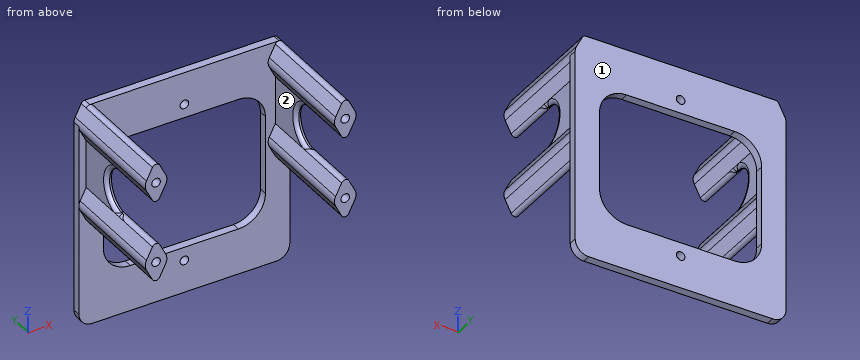
```python
from build123d import *

# Parameters (mm, degrees)
SKETCH1_R             = 1.6
BOSS_EXTRUDE1_DEPTH   = 40
BOSS_EXTRUDE1_2_DEPTH = 40
BOSS_EXTRUDE1_3_DEPTH = 40
BOSS_EXTRUDE1_4_DEPTH = 40
SKETCH2_R             = 1.6
BOSS_EXTRUDE2_DEPTH   = 3
SKETCH4_W             = 2.672170628
SKETCH4_H             = 17.636363636
BOSS_EXTRUDE3_DEPTH   = 20
SKETCH6_R             = 8
CUT_EXTRUDE2_DEPTH    = 99.18617902
FILLET1_R             = 1.5
BOSS_EXTRUDE4_START   = 20
SKETCH7_R             = 1.6
BOSS_EXTRUDE4_DEPTH   = 20


# Read off the part's stored shape, not the designer's step: Mirror2
with BuildPart() as part:
    # Sketch1 → Boss-Extrude1 (new body)
    with BuildSketch(Plane(origin=(0, 0, 0), x_dir=(1, 0, 0), z_dir=(0, 1, 0))):
        with BuildLine():
            Line((-1.336085314, 6.181818182), (-3.562894171, 1.818181818))
            ThreePointArc((-3.562894171, 1.818181818), (-4, 0), (-3.562894171, -1.818181818))
            Line((-3.562894171, -1.818181818), (-1.336085314, -6.181818182))
            ThreePointArc((-1.336085314, -6.181818182), (0, -7), (1.336085314, -6.181818182))
            Line((1.336085314, -6.181818182), (3.562894171, -1.818181818))
            ThreePointArc((3.562894171, -1.818181818), (4, 0), (3.562894171, 1.818181818))
            Line((3.562894171, 1.818181818), (1.336085314, 6.181818182))
            ThreePointArc((1.336085314, 6.181818182), (0, 7), (-1.336085314, 6.181818182))
        make_face()
        with Locations(Location((0, 0, 0), (0, 0, 270))):
            Circle(SKETCH1_R, mode=Mode.SUBTRACT)
    extrude(amount=BOSS_EXTRUDE1_DEPTH)



with BuildPart() as body_2:
    # Sketch1 → Boss-Extrude1 2 (new body)
    with BuildSketch(Plane(origin=(0, 0, 0), x_dir=(1, 0, 0), z_dir=(0, 1, 0))):
        with BuildLine():
            Line((68.663914686, 6.181818182), (66.437105829, 1.818181818))
            ThreePointArc((66.437105829, 1.818181818), (66, 0), (66.437105829, -1.818181818))
            Line((66.437105829, -1.818181818), (68.663914686, -6.181818182))
            ThreePointArc((68.663914686, -6.181818182), (70, -7), (71.336085314, -6.181818182))
            Line((71.336085314, -6.181818182), (73.562894171, -1.818181818))
            ThreePointArc((73.562894171, -1.818181818), (74, 0), (73.562894171, 1.818181818))
            Line((73.562894171, 1.818181818), (71.336085314, 6.181818182))
            ThreePointArc((71.336085314, 6.181818182), (70, 7), (68.663914686, 6.181818182))
        make_face()
        with Locations(Location((70, 0, 0), (0, 0, 270))):
            Circle(SKETCH1_R, mode=Mode.SUBTRACT)
    extrude(amount=BOSS_EXTRUDE1_2_DEPTH)


with BuildPart() as body_3:
    # Sketch1 → Boss-Extrude1 3 (new body)
    with BuildSketch(Plane(origin=(0, 0, 0), x_dir=(1, 0, 0), z_dir=(0, 1, 0))):
        with BuildLine():
            Line((68.663914686, -23.818181818), (66.437105829, -28.181818182))
            ThreePointArc((66.437105829, -28.181818182), (66, -30), (66.437105829, -31.818181818))
            Line((66.437105829, -31.818181818), (68.663914686, -36.181818182))
            ThreePointArc((68.663914686, -36.181818182), (70, -37), (71.336085314, -36.181818182))
            Line((71.336085314, -36.181818182), (73.562894171, -31.818181818))
            ThreePointArc((73.562894171, -31.818181818), (74, -30), (73.562894171, -28.181818182))
            Line((73.562894171, -28.181818182), (71.336085314, -23.818181818))
            ThreePointArc((71.336085314, -23.818181818), (70, -23), (68.663914686, -23.818181818))
        make_face()
        with Locations(Location((70, -30, 0), (0, 0, 270))):
            Circle(SKETCH1_R, mode=Mode.SUBTRACT)
    extrude(amount=BOSS_EXTRUDE1_3_DEPTH)


with BuildPart() as body_4:
    # Sketch1 → Boss-Extrude1 4 (new body)
    with BuildSketch(Plane(origin=(0, 0, 0), x_dir=(1, 0, 0), z_dir=(0, 1, 0))):
        with BuildLine():
            Line((-1.336085314, -23.818181818), (-3.562894171, -28.181818182))
            ThreePointArc((-3.562894171, -28.181818182), (-4, -30), (-3.562894171, -31.818181818))
            Line((-3.562894171, -31.818181818), (-1.336085314, -36.181818182))
            ThreePointArc((-1.336085314, -36.181818182), (0, -37), (1.336085314, -36.181818182))
            Line((1.336085314, -36.181818182), (3.562894171, -31.818181818))
            ThreePointArc((3.562894171, -31.818181818), (4, -30), (3.562894171, -28.181818182))
            Line((3.562894171, -28.181818182), (1.336085314, -23.818181818))
            ThreePointArc((1.336085314, -23.818181818), (0, -23), (-1.336085314, -23.818181818))
        make_face()
        with Locations(Location((0, -30, 0), (0, 0, 270))):
            Circle(SKETCH1_R, mode=Mode.SUBTRACT)
    extrude(amount=BOSS_EXTRUDE1_4_DEPTH)


with BuildPart() as part_1:
    add(part.part)

    add(body_2.part)  # Boss-Extrude2 merges body 2

    add(body_3.part)  # Boss-Extrude2 merges body 3

    add(body_4.part)  # Boss-Extrude2 merges body 4
    # Sketch2 → Boss-Extrude2 (add)
    with BuildSketch(Plane(origin=(0, 40, 0), x_dir=(1, 0, 0), z_dir=(0, 1, 0))):
        with BuildLine():
            Line((1, 46), (69, 46))
            ThreePointArc((69, 46), (72.535533906, 44.535533906), (74, 41))
            Line((74, 41), (74, -30))
            ThreePointArc((74, -30), (73.889188648, -30.934992865), (73.562894171, -31.818181818))
            Line((73.562894171, -31.818181818), (71.336085314, -36.181818182))
            ThreePointArc((71.336085314, -36.181818182), (70.783349452, -36.779204298), (70, -37))
            Line((70, -37), (0, -37))
            ThreePointArc((0, -37), (-0.783349452, -36.779204298), (-1.336085314, -36.181818182))
            Line((-1.336085314, -36.181818182), (-3.562894171, -31.818181818))
            ThreePointArc((-3.562894171, -31.818181818), (-3.889188648, -30.934992865), (-4, -30))
            Line((-4, -30), (-4, 41))
            ThreePointArc((-4, 41), (-2.535533906, 44.535533906), (1, 46))
        make_face()
        with Locations(Location((35, -25, 0), (0, 0, 270))):
            Circle(SKETCH2_R, mode=Mode.SUBTRACT)
        with Locations(Location((35, 34, 0), (0, 0, 270))):
            Circle(SKETCH2_R, mode=Mode.SUBTRACT)
        with BuildLine():
            Line((15, 29), (55, 29))
            ThreePointArc((55, 29), (62.071067812, 26.071067812), (65, 19))
            Line((65, 19), (65, -10))
            ThreePointArc((65, -10), (62.071067812, -17.071067812), (55, -20))
            Line((55, -20), (15, -20))
            ThreePointArc((15, -20), (7.928932188, -17.071067812), (5, -10))
            Line((5, -10), (5, 19))
            ThreePointArc((5, 19), (7.928932188, 26.071067812), (15, 29))
        make_face(mode=Mode.SUBTRACT)
    extrude(amount=BOSS_EXTRUDE2_DEPTH)

    # Sketch4 → Boss-Extrude3 (add)
    with BuildSketch(Plane.XZ.offset(-40)):
        with Locations((0, 15)):
            Rectangle(SKETCH4_W, SKETCH4_H)
    extrude(amount=BOSS_EXTRUDE3_DEPTH)

    # Sketch6 → Cut-Extrude2 (cut, through all)
    with BuildSketch(Plane.ZY.offset(1.336085314)):
        with Locations((15, 20)):
            Circle(SKETCH6_R)
    extrude(amount=-CUT_EXTRUDE2_DEPTH, mode=Mode.SUBTRACT)

    # Fillet1
    # the kernel refuses this fillet: 1.5 mm, written as the material it takes off along each edge
    with BuildSketch(Plane(origin=(1.336085314, 20, 15), x_dir=(0, -0.45244386791178526, 0.8917928831231068), z_dir=(0, -0.8917928831231068, -0.45244386791178526))) as fillet1_piece_1_section:
        with BuildLine():
            CenterArc((8 + FILLET1_R, FILLET1_R), FILLET1_R, 180, 90)
            Line((8, FILLET1_R), (8, 0))
            Line((8, 0), (8 + FILLET1_R, 0))
        make_face()
    fillet1_piece_1 = revolve(axis=Axis((1.336085314, 20, 15), (-1, 0, 0)), revolution_arc=233.801176838, mode=Mode.PRIVATE)
    fillet1_piece_1 = fillet1_piece_1 - Plane(origin=(0, 21.66747918, 5.5), x_dir=(-0.8907235428302468, 0, 0.45454545454545436), z_dir=(0, -1, 0)) * Cylinder(1.5, 38, mode=Mode.PRIVATE)
    fillet1_piece_1 = fillet1_piece_1 - Plane(origin=(0, 21.66747918, 24.5), x_dir=(0.8907235428302462, 0, -0.4545454545454553), z_dir=(0, -1, 0)) * Cylinder(1.5, 38, mode=Mode.PRIVATE)
    add(fillet1_piece_1, mode=Mode.SUBTRACT)
    with BuildSketch(Plane(origin=(-1.336085314, 20, 15), x_dir=(0, -0.45244386791178526, 0.8917928831231068), z_dir=(0, -0.8917928831231068, -0.45244386791178526))) as fillet1_piece_2_section:
        with BuildLine():
            CenterArc((8 + FILLET1_R, -FILLET1_R), FILLET1_R, 90, 90)
            Line((8, -FILLET1_R), (8, 0))
            Line((8, 0), (8 + FILLET1_R, 0))
        make_face()
    fillet1_piece_2 = revolve(axis=Axis((-1.336085314, 20, 15), (-1, 0, 0)), revolution_arc=233.801176838, mode=Mode.PRIVATE)
    fillet1_piece_2 = fillet1_piece_2 - Plane(origin=(0, 21.66746874, 5.5), x_dir=(-0.8907235428302468, 0, 0.45454545454545436), z_dir=(0, -1, 0)) * Cylinder(1.5, 39, mode=Mode.PRIVATE)
    fillet1_piece_2 = fillet1_piece_2 - Plane(origin=(0, 21.66746874, 24.5), x_dir=(0.8907235428302462, 0, -0.4545454545454553), z_dir=(0, -1, 0)) * Cylinder(1.5, 39, mode=Mode.PRIVATE)
    add(fillet1_piece_2, mode=Mode.SUBTRACT)

    # Sketch7 → Boss-Extrude4 (add)
    with BuildSketch(Plane.XZ.offset(-40).offset(BOSS_EXTRUDE4_START)):
        with Locations(Location((0, 30, 0), (0, 0, 270))):
            Circle(SKETCH7_R)
        with Locations(Location((0, 0, 0), (0, 0, 270))):
            Circle(SKETCH7_R)
        with Locations(Location((70, 0, 0), (0, 0, 270))):
            Circle(SKETCH7_R)
        with Locations(Location((70, 30, 0), (0, 0, 270))):
            Circle(SKETCH7_R)
    extrude(amount=-BOSS_EXTRUDE4_DEPTH)

    # Mirror2: part across plane


with BuildPart() as part_2:
    add(part_1.part)
    add(part_1.part.mirror(Plane.ZY.offset(-35)))


solid = part_2.part
```
Here's how the part is built. I have some questions about the finished solid (model axes, mm). Face numbers are marked on the shaded views. Coordinates: 2 decimals unless noted, no trailing zeros. Write each loop counter-clockwise with the first axis right and the second up, starting at its lowest first coordinate (ties: lowest second). Pieces come first, ordered by that corner, then holes. Notation, with made-up numbers: (-38, 87) - (-5, 87) arc R21 ccw to (-5, 117) - close; hole circle Ø11 at (47.5, 40). An arc over 180 degrees is marked (long way). One line per item, written item: value.
1) We'd pull the mould along Z, two halves only. Please class the marked faces 1 and 2: pulls with the +Z half, pulls with the -Z half, needs draft (parallel to the pull), parting line crosses it, or undercut.
Model answer:
face 1: needs draft
face 2: undercut
2) Suppose I cut it at B-B on x = 35. Write out the boundary of the cut face in (y, z), and give its area (3 significant figures).
Model answer:
outline: (40, -46) - (43, -46) - (43, -35.6) - (40, -35.6) - close; (40, -32.4) - (43, -32.4) - (43, -29) - (40, -29) - close; (40, 20) - (43, 20) - (43, 23.4) - (40, 23.4) - close; (40, 26.6) - (43, 26.6) - (43, 37) - (40, 37) - close
area: 82.8 mm²
3) Suppose I cut it at A-A on z = -27. Write out the boundary of the cut face in (x, y), and give its area (3 significant figures).
Model answer:
outline: (-4, 40) - (9, 40) - (9, 43) - (-4, 43) - close; (61, 40) - (74, 40) - (74, 43) - (61, 43) - close
area: 78.0 mm²
4) I'm going to push flat-ended pins straight in: P1, Ø1, axis at y = 25.5, z = 16.5, coming from the +X side; P2, Ø2.5, axis at x = 69.5, z = 0.5, coming from the -Y side; P3, Ø2.5, axis at x = 70, z = 30, coming from the -Y side; P4, Ø10, axis at y = 30.5, z = -7.5, coming from the -X side. Where does each tip first touch, or does it pass through?
Model answer:
P1: passes through
P2: stops at y = 0
P3: stops at y = 20
P4: stops at x = -3.21
5) Suppose I cut it at D-D on x = 6. Write out the boundary of the cut face in (y, z).
Model answer:
outline: (40, -46) - (43, -46) - (43, -23.36) - (40, -23.36) - close; (40, 14.36) - (43, 14.36) - (43, 37) - (40, 37) - close
6) I need wall thicknesses on line 1 along X through (y, z) = (8.25, 30); line 2 along Z through (x, y) = (70, 11.75); line 3 along X through (y, z) = (30, 19.5). Which ranges of each line are inside material? Lowest first, please.
Model answer:
line 1: x = -4 to -1.6, 1.6 to 4, 66 to 68.4, 71.6 to 74
line 2: z = -7 to -1.6, 1.6 to 7, 23 to 28.4, 31.6 to 37
line 3: x = -1.34 to 1.34, 68.66 to 71.34
